```python
from build123d import *

# Parameters (mm, degrees)
SKETCH1_W      = 80
SKETCH1_H      = 80
EXTRUDE1_DEPTH = 20
SKETCH2_W      = 40
SKETCH2_H      = 40
EXTRUDE2_DEPTH = 110
EXTRUDE3_DEPTH = 110


with BuildPart() as part:
    # Sketch1 → Extrude1 (new body)
    with BuildSketch(Plane(origin=(0, 0, 0), x_dir=(1, 0, 0), z_dir=(0, 1, 0))):
        with Locations((-40, 40)):
            Rectangle(SKETCH1_W, SKETCH1_H)
    extrude(amount=EXTRUDE1_DEPTH)

    # Sketch2 → Extrude2 (add)
    with BuildSketch(Plane(origin=(0, 20, 0), x_dir=(1, 0, 0), z_dir=(0, 1, 0))):
        with Locations((-40, 40)):
            Rectangle(SKETCH2_W, SKETCH2_H)
    extrude(amount=EXTRUDE2_DEPTH)

    # Sketch3 → Extrude3 (cut)
    with BuildSketch(Plane.XY.offset(-20)):
        Polygon((-60, 40), (-40, 130), (-60, 130), align=None)
        Polygon((-40, 130), (-20, 40), (-20, 130), align=None)
        Polygon((-50, 40), (-40, 85), (-30, 40), (-30, 30), (-50, 30), align=None)
    extrude(amount=-EXTRUDE3_DEPTH, mode=Mode.SUBTRACT)


solid = part.part
```
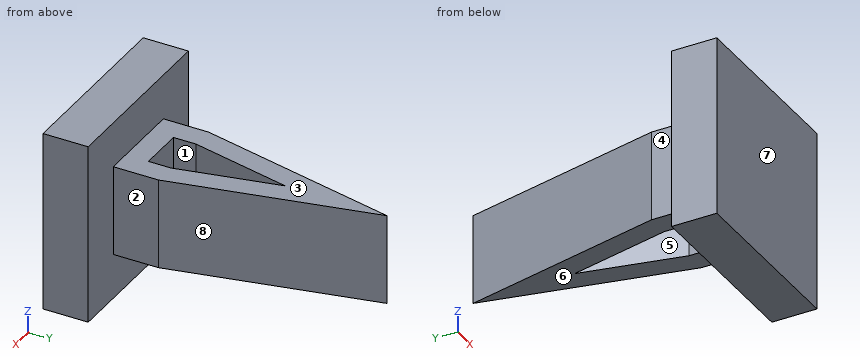
CAD build for the part. Positions are in the model's coordinates, mm. Face numbers are marked on the shaded views. A direction names the side the tool comes from. Round coordinates to 2 decimals unless told otherwise and drop trailing zeros. Loops run counter-clockwise (first coordinate to the right, second up) from the corner with the lowest first, then second, coordinate; pieces in that order, holes last. Notation, with made-up numbers: M 18.5,84.5 L 33.5,84.5 A31 ccw 33.5,118.5 Z; hole C 29,13 d3. An arc over 180 degrees is marked long. Return JSON: item names as keys, results as strings. Group by question number.
(1) Drop flat-ended pins along their axis: P1, Ø10, axis at y = 30, z = -43.5, coming from the -X side; P2, Ø12, axis at y = 54.5, z = -40, coming from the -X side; P3, Ø6, axis at y = 105, z = -20.5, coming from the +X side. Give the stop position or say it passes through.
(2) Saw through at C-C, the plane x = -53.5. List the corners of the cut face in (y, z), and give its area (3 significant figures).
(3) Saw through at D-D, the plane y = 51. List the corners of the cut face in (x, z).
(4) Tool access for the marked faces 1, 2, 3 and 4: list every direction of +Z, -Z, +X, -X, +Y, -Y with a clear straight run to the whole face (end or side of a thin tool).
(5) Saw through at A-A, the plane x = -35. List the corners of the cut face in (y, z), and give its area (3 significant figures).
(6) Saw through at B-B, the plane z = -28.5. List the corners of the cut face in (x, y).
(7) Wall check: probe 1 along Y at (x, z) = (-37, -74); probe 2 along X at (y, z) = (36, -49.5); probe 3 along Z at (x, y) = (-42, 98). Give the ranges that are in metal, low to high. Write a range as [from, to].
(8) Mould opens along Y. For the marked faces 5, 6, 7 and 8 say: +Y half, -Y half, draft (parallel to the pull), parting line (faces both ways), or undercut.
Answer list:
{
 "1": {"P1": "x = -60", "P2": "x = -58.11", "P3": "x = -33.78"},
 "2": {"outline": "M 0,-80 L 20,-80 L 20,-60 L 69.25,-60 L 69.25,-20 L 20,-20 L 20,0 L 0,0 Z", "area": "3,570 mm2"},
 "3": {"outline": "M -57.56,-60 L -47.56,-60 L -47.56,-20 L -57.56,-20 Z; M -32.44,-60 L -22.44,-60 L -22.44,-20 L -32.44,-20 Z"},
 "4": {"face 1": "+Z, -Z", "face 2": "+Z, -Z, +X, +Y", "face 3": "+Z, +X, -X, +Y", "face 4": "+Z, -Z, -X, +Y"},
 "5": {"outline": "M 0,-80 L 20,-80 L 20,-60 L 30,-60 L 30,-20 L 20,-20 L 20,0 L 0,0 Z; M 62.5,-60 L 107.5,-60 L 107.5,-20 L 62.5,-20 Z", "area": "3,800 mm2"},
 "6": {"outline": "M -80,0 L 0,0 L 0,20 L -20,20 L -20,40 L -40,130 L -60,40 L -60,20 L -80,20 Z; hole M -50,30 L -30,30 L -30,40 L -40,85 L -50,40 Z"},
 "7": {"probe 1": "[0, 20]", "probe 2": "[-60, -50], [-30, -20]", "probe 3": "[-60, -20]"},
 "8": {"face 5": "undercut", "face 6": "draft", "face 7": "-Y half", "face 8": "+Y half"}
}
